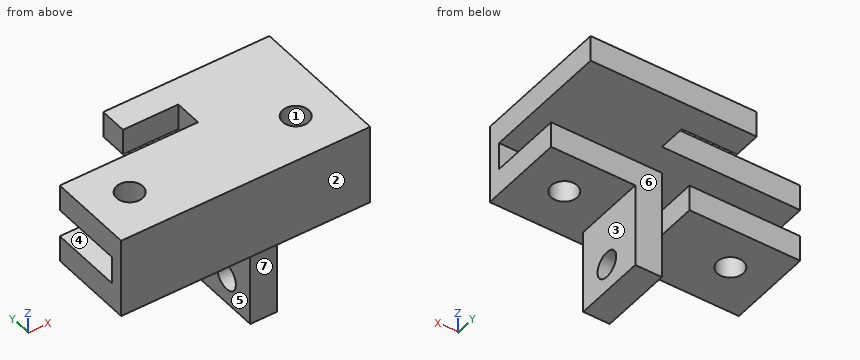
from build123d import *

# Parameters (mm, degrees)
BOSS_EXTRUDE1_DEPTH    = 14.2875
SKETCH4_R              = 1.5
CUT_EXTRUDE1_DEPTH     = 20.646048082
CUT_EXTRUDE3_REACH     = 21.646
SKETCH8_W              = 3.175
SKETCH8_H              = 8.382
SKETCH6_W              = 9.7
SKETCH6_H              = 8.382
SKETCH6_R              = 1.5
BOSS_EXTRUDE4_DEPTH    = 3.048
RIGHT_RAMP_MOUNT_DEPTH = 3


with BuildPart() as part:
    # Sketch2 → Boss-Extrude1 (new, symmetric)
    with BuildSketch(Plane(origin=(0, 0, 0), x_dir=(0, 0, -1), z_dir=(1, 0, 0))):
        Polygon((3, 1.5), (3, 9.882), (0, 9.882), (0, 0), (6.175, 0), (6.175, 1.5), align=None)
        Polygon((6.175, 1.5), (6.175, 0), (9.175, 0), (9.175, 9.882), (6.175, 9.882), align=None)
    extrude(amount=BOSS_EXTRUDE1_DEPTH, both=True)

    # Sketch4 → Cut-Extrude1 (cut, through all)
    with BuildSketch(Plane(origin=(0, 0, 0), x_dir=(-1, 0, 0), z_dir=(0, 0, -1))):
        with Locations(Location((-9.525, 5.31, 0), (0, 0, 180))):
            Circle(SKETCH4_R)
        with Locations(Location((9.525, 5.31, 0), (0, 0, 180))):
            Circle(SKETCH4_R)
    extrude(amount=CUT_EXTRUDE1_DEPTH, mode=Mode.SUBTRACT)

    # Sketch8 → Cut-Extrude3 (cut, up to next)
    with BuildSketch(Plane(origin=(0, 0, -9.175), x_dir=(-1, 0, 0), z_dir=(0, 0, -1)), mode=Mode.PRIVATE) as cut_extrude3_sk1:
        with Locations((0, 5.691)):
            Rectangle(SKETCH8_W, SKETCH8_H)
    cut_extrude3_tool1 = extrude(cut_extrude3_sk1.sketch, amount=-CUT_EXTRUDE3_REACH, mode=Mode.PRIVATE) & part.part
    add(cut_extrude3_tool1.solids().sort_by_distance((0, 5.691, -9.175))[0], mode=Mode.SUBTRACT)

    # Sketch6 → Boss-Extrude4 (add)
    with BuildSketch(Plane(origin=(1.5875, 0, 0), x_dir=(0, 0, -1), z_dir=(1, 0, 0))):
        with Locations((14.025, 5.691)):
            Rectangle(SKETCH6_W, SKETCH6_H)
        with Locations(Location((15.7, 5.31, 0), (0, 0, 180))):
            Circle(SKETCH6_R, mode=Mode.SUBTRACT)
    extrude(amount=BOSS_EXTRUDE4_DEPTH)

    # Sketch9 → Right Ramp Mount (add)
    with BuildSketch(Plane.XY):
        Polygon((1.5785, 9.882), (14.2875, 9.882), (14.2875, 16.232), (-4.7715, 16.232), (-4.7715, 13.057), (1.5785, 13.057), align=None)
    extrude(amount=-RIGHT_RAMP_MOUNT_DEPTH)


solid = part.part
Could you check a few things on this model? Use its own coordinates, in mm. Face numbers are marked on the shaded views. A direction names the side the tool comes from. Give positions to 0.01 mm unless a question says otherwise; leave off trailing zeros. Order: outer loops, then holes, each group sorted by start corner. A loop starts at its lowest first (then second) coordinate and runs counter-clockwise, first axis right, second up. Notation, with made-up numbers: (7.25, 24.5) - (22.25, 24.5) arc R17 ccw to (22.25, 49.5) - close; hole circle Ø5 at (8, 34.5). An arc over 180 degrees is marked (long way). One line per question, with ' | ' between items. Start each with the question number.
Item 1: For the marked faces 4, 5, 6 and 7, which set-ups out of +Z, -Z, +X, -X, +Y, -Y let a thin tool reach every point of the face, with its end or its side?
Item 2: I want a section at C-C on x = -4. Write out the boundary of the cut face in (y, z) (3 decimals), then the cut area to 3 significant figures.
Item 3: I want a section at A-A on z = -15.7. Write out the boundary of the cut face in (x, y), then the cut area to 3 significant figures.
Item 4: I'm going to push flat-ended pins straight in: pin 1 Ø4 at (x, y) = (-9.525, 5.31) entering from -Z (3 decimals); pin 2 Ø1.8 at (x, y) = (-9.525, 5.31) entering from +Z; pin 3 Ø1.5 at (x, z) = (-7.5, -1) entering from +Y; pin 4 Ø2.5 at (y, z) = (15, -1) entering from -X. Where does each tip first touch, or does it pass through?
Item 5: I want a section at D-D on y = 2.25. Write out the boundary of the cut face in (x, z) (1 decimal), then the cut area to 3 significant figures.
Item 6: Thinking about a two-plate mould opening in Y: for the marked faces 1, 2 and 3, which applies, pulls with the +Y half, pulls with the -Y half, needs draft (parallel to the pull), parting line crosses it, or undercut?
Item 7: I need wall thicknesses on probe 1 along X at (y, z) = (5.31, -2) (1 decimal); probe 2 along X at (y, z) = (8.25, -6.75); probe 3 along Z at (x, y) = (-5.25, 2.25) (3 decimals). Which ranges of each line are inside material? Lowest first, please. Write a range as [from, to].
Item 8: I want a section at B-B on y = 5.31. Give the number of separate pieces and of enclosed holes in the cut face, then the cut area to 3 significant figures.
Verdict:
1) face 4: +X, -X, +Y | face 5: -Z, +Y | face 6: -Z, +X, -X, +Y | face 7: -Z, +X, -X, -Y
2) outline: (0, -9.175) - (9.882, -9.175) - (9.882, -6.175) - (1.5, -6.175) - (1.5, -3) - (9.882, -3) - (9.882, 0) - (0, 0) - close; (13.057, -3) - (16.232, -3) - (16.232, 0) - (13.057, 0) - close | area: 73.6 mm^2
3) outline: (1.59, 1.5) - (4.64, 1.5) - (4.64, 3.81) - (1.59, 3.81) - close; (1.59, 6.81) - (4.64, 6.81) - (4.64, 9.88) - (1.59, 9.88) - close | area: 16.4 mm^2
4) pin 1: z = -9.175 | pin 2: through | pin 3: y = 9.88 | pin 4: x = -4.77
5) outline: (-14.3, -9.2) - (-1.6, -9.2) - (-1.6, -6.2) - (-14.3, -6.2) - close; (-14.3, -3) - (14.3, -3) - (14.3, 0) - (-14.3, 0) - close; (1.6, -18.9) - (4.6, -18.9) - (4.6, -9.2) - (14.3, -9.2) - (14.3, -6.2) - (1.6, -6.2) - close | area: 191 mm^2
6) face 1: undercut | face 2: pulls with the -Y half | face 3: needs draft
7) probe 1: [-14.3, -11], [-8, 8], [11, 14.3] | probe 2: [-14.29, -1.59], [1.59, 14.29] | probe 3: [-9.175, -6.175], [-3, 0]
8) separate pieces: 8 | enclosed holes: 0 | area: 146 mm^2
